Model file for the job. Use its own axes, mm. Face numbers are marked on the shaded views. A direction names the side the tool comes from. Coordinates: 2 decimals unless noted, no trailing zeros. Write each loop counter-clockwise with the first axis right and the second up, starting at its lowest first coordinate (ties: lowest second). Pieces come first, ordered by that corner, then holes. Notation, with made-up numbers: (-3.5, 82.25) -> (2.5, 82.25) arc R13 cw to (2.5, 104.25) -> close; hole circle Ø9 at (-11, -12). An arc over 180 degrees is marked (long way). Answer as a JSON object with one key per item and string values. Group by question number.
from build123d import *

# Parameters (mm, degrees)
SKETCH1_R           = 28
BOSS_EXTRUDE1_DEPTH = 38
BOSS_EXTRUDE2_DEPTH = 5.5
SKETCH4_R           = 19.05
CUT_EXTRUDE1_DEPTH  = 2.5
CUT_EXTRUDE2_DEPTH  = 5.5
CIRPATTERN1_COUNT   = 4
BOSS_EXTRUDE3_DEPTH = 9.5
CUT_EXTRUDE3_DEPTH  = 9.5
CIRPATTERN2_COUNT   = 4
SKETCH8_R           = 20
BOSS_EXTRUDE4_DEPTH = 2.5
SKETCH9_R           = 7.5
BOSS_EXTRUDE5_DEPTH = 1
SKETCH10_R          = 7
BOSS_EXTRUDE6_DEPTH = 30
SKETCH11_R          = 2
CUT_EXTRUDE4_DEPTH  = 10
CUT_EXTRUDE5_DEPTH  = 60
CIRPATTERN3_COUNT   = 4


with BuildPart() as part:
    # Sketch1 → Boss-Extrude1 (new body)
    with BuildSketch(Plane(origin=(0, 0, 0), x_dir=(0, 0, -1), z_dir=(1, 0, 0))):
        Circle(SKETCH1_R)
    extrude(amount=BOSS_EXTRUDE1_DEPTH)

    # Sketch2 → Boss-Extrude2 (add)
    with BuildSketch(Plane(origin=(38, 0, 0), x_dir=(0, 0, -1), z_dir=(1, 0, 0))):
        Polygon((28.5, 0), (28.5, 28.5), (-28.5, 28.5), (-28.5, -28.5), (28.5, -28.5), align=None)
    extrude(amount=BOSS_EXTRUDE2_DEPTH)

    # Sketch4 → Cut-Extrude1 (cut)
    with BuildSketch(Plane(origin=(43.5, 0, 0), x_dir=(0, 0, -1), z_dir=(1, 0, 0))):
        Circle(SKETCH4_R)
    extrude(amount=-CUT_EXTRUDE1_DEPTH, mode=Mode.SUBTRACT)

    # Sketch5 → Cut-Extrude2 (cut)
    with BuildSketch(Plane(origin=(43.5, 0, 0), x_dir=(0, 0, -1), z_dir=(1, 0, 0))):
        Polygon((-27.085786438, 28.5), (-28.5, 27.085786438), (-28.5, 28.5), align=None)
    cut_extrude2 = extrude(amount=-CUT_EXTRUDE2_DEPTH, mode=Mode.SUBTRACT)

    # CirPattern1: Cut-Extrude2 ×4 about axis
    cirpattern1_axis = Axis((0, 0, 0), (1, 0, 0))
    for i in range(1, CIRPATTERN1_COUNT):
        add(cut_extrude2.rotate(cirpattern1_axis, i * 360 / CIRPATTERN1_COUNT), mode=Mode.SUBTRACT)

    # Sketch6 → Boss-Extrude3 (add)
    with BuildSketch(Plane.ZY):
        Polygon((28.5, 0), (28.5, -28.5), (-28.5, -28.5), (-28.5, 28.5), (28.5, 28.5), align=None)
    extrude(amount=BOSS_EXTRUDE3_DEPTH)

    # Sketch7 → Cut-Extrude3 (cut)
    with BuildSketch(Plane.ZY.offset(9.5)):
        Polygon((-24.964466094, 28.5), (-28.5, 24.964466094), (-28.5, 28.5), align=None)
    cut_extrude3 = extrude(amount=-CUT_EXTRUDE3_DEPTH, mode=Mode.SUBTRACT)

    # CirPattern2: Cut-Extrude3 ×4 about axis
    cirpattern2_axis = Axis((0, 0, 0), (1, 0, 0))
    for i in range(1, CIRPATTERN2_COUNT):
        add(cut_extrude3.rotate(cirpattern2_axis, i * 360 / CIRPATTERN2_COUNT), mode=Mode.SUBTRACT)

    # Sketch8 → Boss-Extrude4 (add)
    with BuildSketch(Plane.ZY.offset(9.5)):
        Circle(SKETCH8_R)
    extrude(amount=BOSS_EXTRUDE4_DEPTH)

    # Sketch9 → Boss-Extrude5 (add)
    with BuildSketch(Plane.ZY.offset(12)):
        Circle(SKETCH9_R)
    extrude(amount=BOSS_EXTRUDE5_DEPTH)

    # Sketch10 → Boss-Extrude6 (add)
    with BuildSketch(Plane.ZY.offset(13)):
        Circle(SKETCH10_R)
    extrude(amount=BOSS_EXTRUDE6_DEPTH)

    # Sketch11 → Cut-Extrude4 (cut)
    with BuildSketch(Plane.ZY.offset(43)):
        Circle(SKETCH11_R)
    extrude(amount=-CUT_EXTRUDE4_DEPTH, mode=Mode.SUBTRACT)

    # Sketch12 → Cut-Extrude5 (cut)
    with BuildSketch(Plane(origin=(43.5, 0, 0), x_dir=(0, 0, -1), z_dir=(1, 0, 0))):
        with BuildLine():
            ThreePointArc((-23.5, 20.75), (-21.555456352, 21.555456352), (-20.75, 23.5))
            Line((-20.75, 23.5), (-23.5, 23.5))
            Line((-23.5, 23.5), (-23.5, 20.75))
        make_face()
        with BuildLine():
            Line((-23.5, 23.5), (-20.75, 23.5))
            ThreePointArc((-20.75, 23.5), (-25.444543648, 25.444543648), (-23.5, 20.75))
            Line((-23.5, 20.75), (-23.5, 23.5))
        make_face()
    cut_extrude5 = extrude(amount=-CUT_EXTRUDE5_DEPTH, mode=Mode.SUBTRACT)

    # CirPattern3: Cut-Extrude5 ×4 about axis
    cirpattern3_axis = Axis((0, 0, 0), (1, 0, 0))
    for i in range(1, CIRPATTERN3_COUNT):
        add(cut_extrude5.rotate(cirpattern3_axis, i * 360 / CIRPATTERN3_COUNT), mode=Mode.SUBTRACT)


solid = part.part
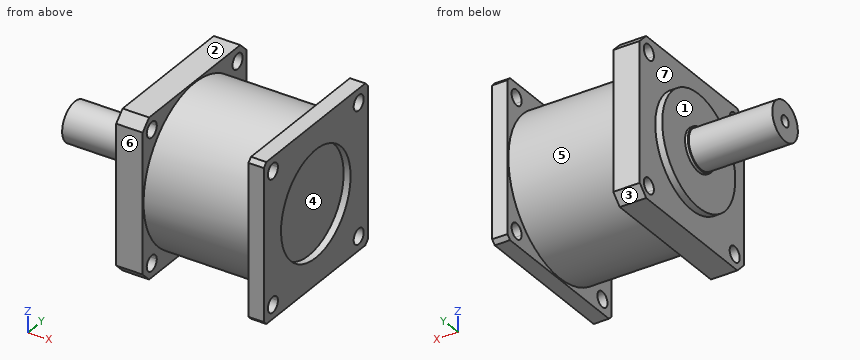
(1) Cut at C-C on y = -22.5. List the corners of the cut face in (x, z), plus the area to 3 significant figures.
(2) Pin check, flat tips, straight feed: pin 1 (9 mm diameter, centred on y = -23.5, z = -23.5, fed in from -X); pin 2 (3 mm diameter, centred on y = 5, z = -12.5, fed in from -X); pin 3 (1.5 mm diameter, centred on y = 6, z = -10.5, fed in from +X). Stop position of each tip, or through.
(3) 3-axis set-ups, long thin cutter, end or side, ignore diameter. For the marked faces 1, 2 and 3: which of +Z, -Z, +X, -X, +Y, -Y reach the whole face in a straight line?
(4) Wall check: probe 1 along X at (y, z) = (-20, 23); probe 2 along X at (y, z) = (-10, -8); probe 3 along Z at (x, y) = (-6, -23). Give the ranges that are in metal, low to high.
(5) Pull direction X, two halves, no side cores. Call the marked faces 4, 5, 6 and 7: released by +X, released by -X, zero draft, split by the parting line, or undercut.
(6) Cut at D-D on z = 14.5. List the corners of the cut face in (x, y).
Results found:
{
 "1": {"outline": "(-9.5, -28.5) -> (0, -28.5) -> (0, -26.06) -> (-9.5, -26.06) -> close; (-9.5, -20.94) -> (0, -20.94) -> (0, -16.67) -> (38, -16.67) -> (38, -20.94) -> (43.5, -20.94) -> (43.5, 20.94) -> (38, 20.94) -> (38, 16.67) -> (0, 16.67) -> (0, 20.94) -> (-9.5, 20.94) -> close; (-9.5, 26.06) -> (0, 26.06) -> (0, 28.5) -> (-9.5, 28.5) -> close; (38, -28.5) -> (43.5, -28.5) -> (43.5, -26.06) -> (38, -26.06) -> close; (38, 26.06) -> (43.5, 26.06) -> (43.5, 28.5) -> (38, 28.5) -> close", "area": "1,970 mm²"},
 "2": {"pin 1": "stops at x = -9.5", "pin 2": "stops at x = -12", "pin 3": "stops at x = 41"},
 "3": {"face 1": "-X", "face 2": "+Z, +X, -X, +Y, -Y", "face 3": "-Z, -X, +Y"},
 "4": {"probe 1": "x = -9.5 to 0, 38 to 43.5", "probe 2": "x = -12 to 41", "probe 3": "z = -28.5 to -26.2, -20.8 to 20.8, 26.2 to 28.5"},
 "5": {"face 4": "released by +X", "face 5": "undercut", "face 6": "zero draft", "face 7": "released by -X"},
 "6": {"outline": "(-12, -13.77) -> (-9.5, -13.77) -> (-9.5, -28.5) -> (0, -28.5) -> (0, -23.95) -> (38, -23.95) -> (38, -28.5) -> (43.5, -28.5) -> (43.5, -12.36) -> (41, -12.36) -> (41, 12.36) -> (43.5, 12.36) -> (43.5, 28.5) -> (38, 28.5) -> (38, 23.95) -> (0, 23.95) -> (0, 28.5) -> (-9.5, 28.5) -> (-9.5, 13.77) -> (-12, 13.77) -> close"}
}
